Can you work these out from the drawing? Everything is in mm from the part's minimum corner. A direction names the side the tool comes from. Coordinates: 2 decimals unless noted, no trailing zeros. Loops run counter-clockwise (first coordinate to the right, second up) from the corner with the lowest first, then second, coordinate; pieces in that order, holes last. Notation, with made-up numbers: (17, 25.25) - (57, 25.25) arc R29 ccw to (57, 62.25) - close; hole circle Ø11 at (-32, -7.5). An arc over 180 degrees is marked (long way). Use CSV: the item, a comma, the result in double quotes.
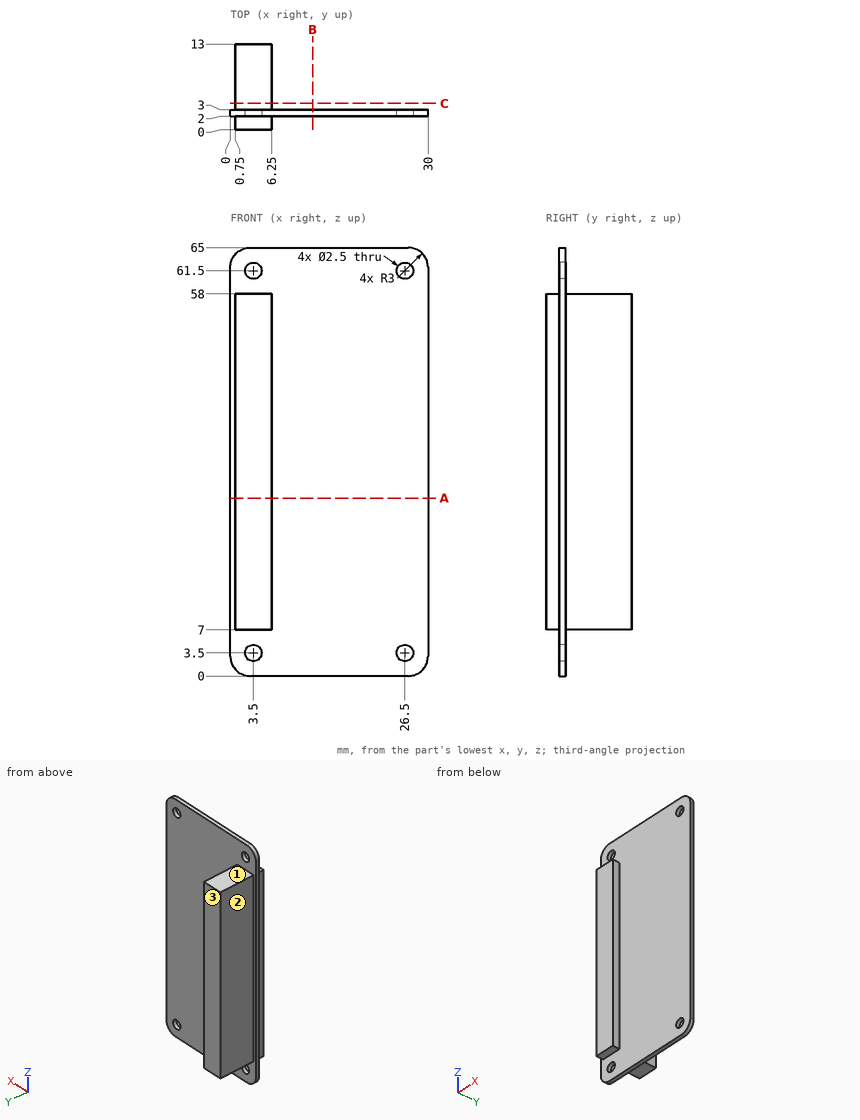
(1) Which directions (+Z, -Z, +X, -X, +Y, -Y) give clear straight access to the entire face, cutting with the end or side of a thin tool? Please do the marked faces 1, 2 and 3.
Computed:
face 1,"+Z, +X, -X, +Y"
face 2,"+Z, -Z, -X, +Y"
face 3,"+Z, -Z, +X, -X, +Y"
(2) Suppose I cut it at B-B (x = 12.5). Write out the boundary of the cut face in (y, z).
Computed:
outline,"(2, 0) - (3, 0) - (3, 65) - (2, 65) - close"
(3) Suppose I cut it at A-A (z = 27). Write out the boundary of the cut face in (x, y).
Computed:
outline,"(0, 2) - (0.75, 2) - (0.75, 0) - (6.25, 0) - (6.25, 2) - (30, 2) - (30, 3) - (6.25, 3) - (6.25, 13) - (0.75, 13) - (0.75, 3) - (0, 3) - close"
(4) Suppose I cut it at C-C (y = 4). Write out the boundary of the cut face in (x, z), plus the area to 4 significant figures.
Computed:
outline,"(0.75, 7) - (6.25, 7) - (6.25, 58) - (0.75, 58) - close"
area,"280.5 mm²"
(5) Will these pins go through, and if not, where does the flat tip stop? pin 1 (4 mm diameter, centred on x = 12, z = 46.5, fed in from +Y); pin 2 (1 mm diameter, centred on y = 1, z = 30, fed in from +X); pin 3 (5 mm diameter, centred on x = 8, y = 8.5, fed in from -Z); pin 4 (3 mm diameter, centred on y = 4, z = 51.5, fed in from +X).
Computed:
pin 1,"stops at y = 3"
pin 2,"stops at x = 6.25"
pin 3,"stops at z = 7"
pin 4,"stops at x = 30"
(6) Please list where these lines run through material, in increasing order: line 1 (Z direction, x = 26.5, y = 2.5); line 2 (Y direction, x = 10, z = 46); line 3 (X direction, y = 5.5, z = 55).
Computed:
line 1,"z = 0 to 2.25, 4.75 to 60.25, 62.75 to 65"
line 2,"y = 2 to 3"
line 3,"x = 0.75 to 6.25"
